Geometry check sheet. Reference: the model listing, model coordinates, mm. A direction names the side the tool comes from. Give positions to 0.01 mm unless a question says otherwise; leave off trailing zeros. Order: outer loops, then holes, each group sorted by start corner. A loop starts at its lowest first (then second) coordinate and runs counter-clockwise, first axis right, second up.
from build123d import *

# Parameters (mm, degrees)
SKETCH1_W           = 110
SKETCH1_H           = 35
BOSS_EXTRUDE1_DEPTH = 20
SKETCH2_R           = 2
BOSS_EXTRUDE2_DEPTH = 20


with BuildPart() as part:
    # Sketch1 → Boss-Extrude1 (new body)
    with BuildSketch(Plane(origin=(0, 0, 0), x_dir=(1, 0, 0), z_dir=(0, 1, 0))):
        with Locations((55, 17.5)):
            Rectangle(SKETCH1_W, SKETCH1_H)
    extrude(amount=BOSS_EXTRUDE1_DEPTH)

    # Sketch2 → Boss-Extrude2 (add)
    with BuildSketch(Plane.ZY):
        with Locations(Location((-31, 17.5, 0), (0, 0, 180))):
            Circle(SKETCH2_R)
        with Locations(Location((-31, 2.5, 0), (0, 0, 180))):
            Circle(SKETCH2_R)
    extrude(amount=BOSS_EXTRUDE2_DEPTH)


solid = part.part
Item 1: Draft check along Y on faces 1 (the cylindrical face through (-9.86, 3.266, -32.847)), 2 (the flat face through (54, 0, -18)), 3 (the flat face through (54, 20, -18)). Enter one of: released by +Y, released by -Y, zero draft, split by the parting line, or undercut.
Reported:
face 1: undercut
face 2: released by -Y
face 3: released by +Y
Item 2: Gauge pin test, flat ends, axial feed: pin 1 (5 mm diameter, centred on x = 60, z = -26, fed in from -Y); pin 2 (3 mm diameter, centred on y = 8.5, z = -15.5, fed in from -X). Record the tip position at first contact, or that the pin passes through.
Reported:
pin 1: stops at y = 0
pin 2: stops at x = 0
Item 3: Set-up check for faces 4 (the flat face through (54, 10, -35)), 5 (the cylindrical face through (-9.86, 16.899, -32.908)): record each of +Z, -Z, +X, -X, +Y, -Y from which the full face is reachable in a straight line by a thin tool's end or side.
Reported:
face 4: -Z, +X, -X, +Y, -Y
face 5: -X
Item 4: Sectioned sample at B-B (z = -31). Enter the section's corners in (x, y).
Reported:
outline: (-20, 0.5) - (0, 0.5) - (0, 0) - (110, 0) - (110, 20) - (0, 20) - (0, 19.5) - (-20, 19.5) - (-20, 15.5) - (0, 15.5) - (0, 4.5) - (-20, 4.5) - close
Item 5: Scan lines: L1, parallel to X at y = 7, z = -1.5; L2, parallel to Z at x = -4.5, y = 3.5. Record each from-to range of solid material in increasing order.
Reported:
L1: x = 0 to 110
L2: z = -32.73 to -29.27
Item 6: Sectioned sample at A-A (y = 17.5). Enter the section's corners in (x, z).
Reported:
outline: (-20, -33) - (0, -33) - (0, -35) - (110, -35) - (110, 0) - (0, 0) - (0, -29) - (-20, -29) - close
Item 7: Sectioned sample at C-C (z = -10.5). Enter the section's corners in (x, y), and give its area (3 significant figures).
Reported:
outline: (0, 0) - (110, 0) - (110, 20) - (0, 20) - close
area: 2,200 mm2
